The listing builds one solid part. Answer for the finished solid, in the listing's coordinates (mm). A direction names the side the tool comes from. Round coordinates to 2 decimals unless told otherwise and drop trailing zeros. Loops run counter-clockwise (first coordinate to the right, second up) from the corner with the lowest first, then second, coordinate; pieces in that order, holes last. Notation, with made-up numbers: (-39.75, 89.5) -> (-15.75, 89.5) arc R17 ccw to (-15.75, 110.5) -> close; hole circle Ø9 at (-21, 50.5). An arc over 180 degrees is marked (long way). One line per question, with ' | ' between items.
from build123d import *

# Parameters (mm, degrees)
SKETCH_1_R           = 8
EXTRUDE_1_DEPTH      = 630
SKETCH_3_OUTSIDE_W   = 144.082
SKETCH_3_OUTSIDE_H   = 144.082
SKETCH_3_OUTSIDE_W_2 = 20
SKETCH_3_OUTSIDE_H_2 = 10
CUT_EXTRUDE_2_DEPTH  = 20
SKETCH_4_R           = 4
CUT_EXTRUDE_3_DEPTH  = 14


with BuildPart() as part:
    # 草图1 → 凸台-拉伸1 (new body)
    with BuildSketch(Plane(origin=(0, 0, 0), x_dir=(0, 0, -1), z_dir=(1, 0, 0))):
        Circle(SKETCH_1_R)
    extrude(amount=EXTRUDE_1_DEPTH)

    # 草图3 outside → 切除-拉伸2 (cut)
    with BuildSketch(Plane.ZY):
        Rectangle(SKETCH_3_OUTSIDE_W, SKETCH_3_OUTSIDE_H)
        Rectangle(SKETCH_3_OUTSIDE_W_2, SKETCH_3_OUTSIDE_H_2, mode=Mode.SUBTRACT)
    extrude(amount=-CUT_EXTRUDE_2_DEPTH, mode=Mode.SUBTRACT)

    # 草图4 → 切除-拉伸3 (cut, through all)
    with BuildSketch(Plane(origin=(0, 5, 0), x_dir=(1, 0, 0), z_dir=(0, 1, 0))):
        with Locations((10, 0)):
            Circle(SKETCH_4_R)
    extrude(amount=-CUT_EXTRUDE_3_DEPTH, mode=Mode.SUBTRACT)


solid = part.part
Q1. A cutting plane is placed at A-A on z = 0. Give the vertices of the cut face in (x, y).
Numbers:
outline: (0, -5) -> (6, -5) -> (6, 5) -> (0, 5) -> close; (14, -5) -> (20, -5) -> (20, -8) -> (630, -8) -> (630, 8) -> (20, 8) -> (20, 5) -> (14, 5) -> close
Q2. Find the intervals of material crossed by line 1 (X direction, y = -3.5, z = -0.25); line 2 (Z direction, x = 10, y = -0.5); line 3 (Y direction, x = 293.5, z = 1.25), in increasing order. Write a range as from..to.
Numbers:
line 1: 0..6.01, 13.99..630 | line 2: -7.98..-4, 4..7.98 | line 3: -7.9..7.9
Q3. For faces 1 (the face through (9.9, 5, -4.3)), 2 (the face through (0, 0, 0)), 3 (the face through (9.9, -5, -4.3)), determine the directions among +Z, -Z, +X, -X, +Y, -Y from which every point of the face is accessible in a straight line to the end or side of a thin tool.
Numbers:
face 1: +Z, -Z, -X, +Y | face 2: +Z, -Z, -X, +Y, -Y | face 3: +Z, -Z, -X, -Y
Q4. Given pin 1 Ø3 at (y, z) = (0.5, 5.5) entering from -X; pin 2 Ø3.5 at (y, z) = (-7, 1) entering from -X, each flat-ended and moving along its own axis, determine where each tip first touches the part or whether it passes through.
Numbers:
pin 1: x = 0 | pin 2: x = 20
Q5. A cutting plane is placed at B-B on x = 318.5. Give the vertices of the cut face in (y, z).
Numbers:
outline: circle Ø16 at (0, 0)
